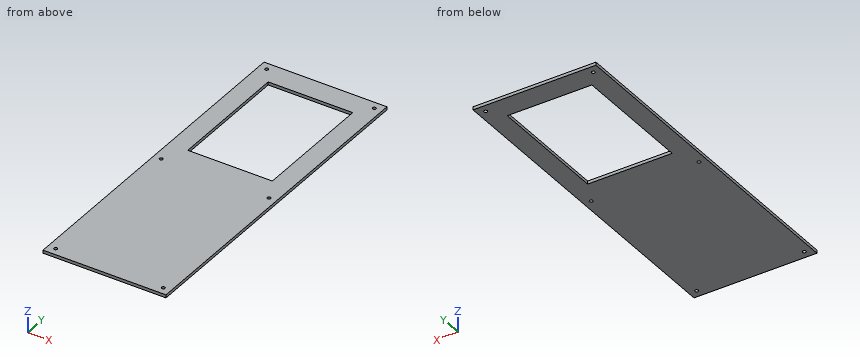
```python
from build123d import *

# Parameters (mm, degrees)
ESQUISSE1_W        = 160
ESQUISSE1_H        = 440
ESQUISSE1_R        = 2.2
ESQUISSE1_W_2      = 110
ESQUISSE1_H_2      = 160
BOSS_EXTRU_1_DEPTH = 4


with BuildPart() as part:
    # Esquisse1 → Boss.-Extru.1 (new body)
    with BuildSketch(Plane.XY):
        Rectangle(ESQUISSE1_W, ESQUISSE1_H)
        with Locations((70, 0)):
            Circle(ESQUISSE1_R, mode=Mode.SUBTRACT)
        with Locations((70, 210)):
            Circle(ESQUISSE1_R, mode=Mode.SUBTRACT)
        with Locations((70, -210)):
            Circle(ESQUISSE1_R, mode=Mode.SUBTRACT)
        with Locations((-70, 210)):
            Circle(ESQUISSE1_R, mode=Mode.SUBTRACT)
        with Locations((-70, 0)):
            Circle(ESQUISSE1_R, mode=Mode.SUBTRACT)
        with Locations((-70, -210)):
            Circle(ESQUISSE1_R, mode=Mode.SUBTRACT)
        with Locations((0, 110)):
            Rectangle(ESQUISSE1_W_2, ESQUISSE1_H_2, mode=Mode.SUBTRACT)
    extrude(amount=BOSS_EXTRU_1_DEPTH)


solid = part.part
```
For this review, take the finished solid that the model builds, in its own axes (mm). Coordinates: 2 decimals unless noted, no trailing zeros. Order: outer loops, then holes, each group sorted by start corner. A loop starts at its lowest first (then second) coordinate and runs counter-clockwise, first axis right, second up. Notation, with made-up numbers: (73, -39.5) - (92, -39.5) arc R35 ccw to (92, -6.5) - close; hole circle Ø3 at (38, 78.5). An arc over 180 degrees is marked (long way). Answer as a JSON object with one key per item and string values. Group by question number.
1. For probe 1 along Y at (x, z) = (70, 0.9); probe 2 along X at (y, z) = (-210, 2); probe 3 along X at (y, z) = (0.5, 2.3), list the stretches that pass through material, from the lowest coordinate up.
2. We need section A-A on x = -36. State the section outline as (y, z) points, then the cut area to 3 significant figures.
3. Clearance check with a flat-ended pin moving along its axis: P1, Ø2.5, axis at x = 70, y = -210, coming from the +Z side. State where the tip first meets the part, or that it passes through.
4. We need section B-B on z = 2.5. State the section outline as (x, y) points, then the cut area to 3 significant figures.
Final values:
{
 "1": {"probe 1": "-220 to -212.2, -207.8 to -2.2, 2.2 to 207.8, 212.2 to 220", "probe 2": "-80 to -72.2, -67.8 to 67.8, 72.2 to 80", "probe 3": "-80 to -72.14, -67.86 to 67.86, 72.14 to 80"},
 "2": {"outline": "(-220, 0) - (30, 0) - (30, 4) - (-220, 4) - close; (190, 0) - (220, 0) - (220, 4) - (190, 4) - close", "area": "1,120 mm²"},
 "3": {"P1": "through"},
 "4": {"outline": "(-80, -220) - (80, -220) - (80, 220) - (-80, 220) - close; hole circle Ø4.4 at (-70, -210); hole circle Ø4.4 at (-70, 0); hole circle Ø4.4 at (-70, 210); hole (-55, 30) - (55, 30) - (55, 190) - (-55, 190) - close; hole circle Ø4.4 at (70, -210); hole circle Ø4.4 at (70, 0); hole circle Ø4.4 at (70, 210)", "area": "52,700 mm²"}
}
